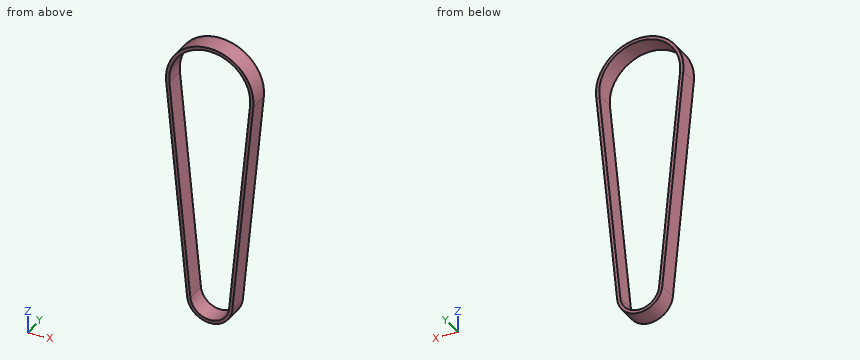
Autodesk Inventor part; units mm, degrees
ref_plane "YZ Plane" through (0, 0, 0) normal (1, 0, 0) x (0, 1, 0)
ref_plane "XZ Plane" through (0, 0, 0) normal (0, 1, 0) x (-1, 0, 0)
ref_plane "XY Plane" through (0, 0, 0) normal (0, 0, 1) x (1, 0, 0)
sketch "Sketch1" plane through (0, 0, 0) normal (0, 1, 0) x (-1, 0, 0)
  line L0 (0, -23.2452) -> (0, 23.2452) construction
  line L1 (0, -34) -> (0, 34) construction
  arc A0 (12.4428, 32.8051) -> (-12.4428, 32.8051) centre (0, 34) ccw
  arc A1 (-5.9725, -34.5735) -> (5.9725, -34.5735) centre (0, -34) ccw
  line L2 (-12.4428, 32.8051) -> (-5.9725, -34.5735)
  line L3 (5.9725, -34.5735) -> (12.4428, 32.8051)
  arc A2 (13.4382, 32.7096) -> (-13.4382, 32.7096) centre (0, 34) ccw
  line L4 (13.4382, 32.7096) -> (6.9679, -34.6691)
  arc A3 (-6.9679, -34.6691) -> (6.9679, -34.6691) centre (0, -34) ccw
  line L5 (-6.9679, -34.6691) -> (-13.4382, 32.7096)
  point P0 (0, 0)
  dimension "d5" = 25
  dimension "d6" = 12
  dimension "d7" = 68
  dimension "d8" = 1
extrude "Extrusion1" add sketch "Sketch1" along normal blind 6
properties part number "Z Axis Belt" material "Rubber"
Here's how the part is built. I have some questions about the finished solid (model axes, mm). Give positions to 0.01 mm unless a question says otherwise; leave off trailing zeros. Loops run counter-clockwise (first coordinate to the right, second up) from the corner with the lowest first, then second, coordinate; pieces in that order, holes last. Notation, with made-up numbers: M -24.5,40 L 28.5,40 A27 ccw 28.5,59 Z; hole C 55.25,35.25 d4. An arc over 180 degrees is marked long. Return JSON: item names as keys, results as strings.
Item 1: Imagine slicing it at B-B on z = 34. List the corners of the cut face in (x, y) for me, then the cut area to 3 significant figures.
A:
{"outline": "M -13.5,0 L -12.5,0 L -12.5,6 L -13.5,6 Z; M 12.5,0 L 13.5,0 L 13.5,6 L 12.5,6 Z", "area": "12.0 mm^2"}
Item 2: Imagine slicing it at C-C on y = 2.8. List the corners of the cut face in (x, z) for me, then the cut area to 3 significant figures.
A:
{"outline": "M -13.44,32.71 L -6.97,-34.67 A7 ccw 6.97,-34.67 L 13.44,32.71 A13.5 ccw long Z; hole M -12.44,32.81 L -5.97,-34.57 A6 ccw 5.97,-34.57 L 12.44,32.81 A12.5 ccw long Z", "area": "198 mm^2"}
Item 3: I'm going to push a flat-ended pin straight in: pin 1 Ø2 at (x, y) = (9.5, 2) entering from +Z. Where does the tip first touch, or does it pass through?
A:
{"pin 1": "stops at z = 44.49"}
Item 4: Please list where these lines run through material, in increasing order: line 1 (X direction, y = 1.8, z = 34); line 2 (X direction, y = 0.55, z = 29); line 3 (Z direction, x = 0.5, y = 0.3).
A:
{"line 1": "x = -13.5 to -12.5, 12.5 to 13.5", "line 2": "x = -13.08 to -12.08, 12.08 to 13.08", "line 3": "z = -40.98 to -39.98, 46.49 to 47.49"}
Item 5: Imagine slicing it at A-A on x = 0. List the corners of the cut face in (y, z) for me.
A:
{"outline": "M 0,-41 L 6,-41 L 6,-40 L 0,-40 Z; M 0,46.5 L 6,46.5 L 6,47.5 L 0,47.5 Z"}
